from build123d import *

# Parameters (mm, degrees)
DODANIE_WYCI_GNI_CIE1_DEPTH = 26.5
SZKIC2_W                    = 110
SZKIC2_H                    = 20.5
WYTNIJ_WYCI_GNI_CIE1_DEPTH  = 30
SZKIC4_W                    = 20.5
SZKIC4_H                    = 25
WYTNIJ_WYCI_GNI_CIE3_DEPTH  = 3
SZKIC5_R                    = 1.6
WYTNIJ_WYCI_GNI_CIE4_DEPTH  = 135.815614823
FILLET1_R                   = 3


with BuildPart() as part:
    # Szkic1 → Dodanie-wyciągnięcie1 (new body)
    with BuildSketch(Plane.XY):
        Polygon((0, 0), (116, 0), (116, 28), (128, 28), (128, 33), (-12, 33), (-12, 28), (0, 28), align=None)
    extrude(amount=DODANIE_WYCI_GNI_CIE1_DEPTH)

    # Szkic2 → Wytnij-wyciągnięcie1 (cut)
    with BuildSketch(Plane(origin=(0, 33, 0), x_dir=(1, 0, 0), z_dir=(0, 1, 0))):
        with Locations((58, -13.25)):
            Rectangle(SZKIC2_W, SZKIC2_H)
    extrude(amount=-WYTNIJ_WYCI_GNI_CIE1_DEPTH, mode=Mode.SUBTRACT)

    # Szkic4 → Wytnij-wyciągnięcie3 (cut)
    with BuildSketch(Plane.ZY):
        with Locations((13.25, 15.5)):
            Rectangle(SZKIC4_W, SZKIC4_H)
    extrude(amount=-WYTNIJ_WYCI_GNI_CIE3_DEPTH, mode=Mode.SUBTRACT)

    # Szkic5 → Wytnij-wyciągnięcie4 (cut, through all)
    with BuildSketch(Plane(origin=(0, 33, 0), x_dir=(1, 0, 0), z_dir=(0, 1, 0))):
        with Locations(Location((-7, -5, 0), (0, 0, 180))):
            Circle(SZKIC5_R)
        with Locations(Location((123, -5, 0), (0, 0, 180))):
            Circle(SZKIC5_R)
        with Locations(Location((123, -21.5, 0), (0, 0, 180))):
            Circle(SZKIC5_R)
        with Locations(Location((-7, -21.5, 0), (0, 0, 180))):
            Circle(SZKIC5_R)
    extrude(amount=-WYTNIJ_WYCI_GNI_CIE4_DEPTH, mode=Mode.SUBTRACT)

    # Fillet1
    fillet1_edges = [part.edges().sort_by_distance(p)[0] for p in [
        (128, 30.5, 26.5),
        (-12, 30.5, 26.5),
        (-12, 30.5, 0),
        (128, 30.5, 0),
    ]]
    fillet(fillet1_edges, radius=FILLET1_R)


solid = part.part
Input: part model. Units: mm. Frame: model coordinates. A direction names the side the tool comes from. Give positions to 0.01 mm unless a question says otherwise; leave off trailing zeros. Write each loop counter-clockwise with the first axis right and the second up, starting at its lowest first coordinate (ties: lowest second). Pieces come first, ordered by that corner, then holes.
Q1. First-contact query: P1, Ø4, axis at x = 123, z = 5, coming from the +Y side; P2, Ø3.5, axis at x = 124, z = 17, coming from the -Y side; P3, Ø8, axis at y = 7.5, z = 10, coming from the -X side; P4, Ø12, axis at y = 5, z = 5.5, coming from the +X side. Flat tips, straight axial feed; report the tip coordinate or a pass-through.
Q2. Section A-A, the plane x = -7. Output: boundary loops of the cut face in (y, z).
Q3. Material intervals for probe 1 along Z at (x, y) = (-7, 30.6); probe 2 along Z at (x, y) = (41.5, 29.5); probe 3 along Y at (x, z) = (83.5, 7.5), sorted ascending.
Q4. Section D-D, the plane x = 105. Output: boundary loops of the cut face in (y, z), plus the area to 4 significant figures.
Q5. Section B-B, the plane z = 17. Output: boundary loops of the cut face in (x, y).
Q6. Set-up query: faces 1 (the face through (127.1, 30.54, 0.86)), 2 (the face through (116, 14, 13)), 3 (the face through (0, 2.7, 14.2)), 4 (the face through (-5, 28, 13)), 5 (the face through (57, 17, 0)). Return all of +Z, -Z, +X, -X, +Y, -Y with unobstructed straight access to the full face (end or side cutting, diameter ignored); none if empty.
Q7. Pull-direction query (X, two-part tool) for faces 6 (the face through (57, 17, 26.5)), 7 (the face through (3, 31, 13)), 8 (the face through (128, 30, 13)); classes: pulls with the +X half, pulls with the -X half, needs draft (parallel to the pull), parting line crosses it, or undercut.
Q8. Section C-C, the plane y = 13. Output: boundary loops of the cut face in (x, z).
Filled in:
1. P1: stops at y = 33
1. P2: stops at y = 28
1. P3: stops at x = 113
1. P4: stops at x = 116
2. outline: (28, 0) - (33, 0) - (33, 3.4) - (28, 3.4) - close; (28, 6.6) - (33, 6.6) - (33, 19.9) - (28, 19.9) - close; (28, 23.1) - (33, 23.1) - (33, 26.5) - (28, 26.5) - close
3. probe 1: z = 0 to 3.4, 6.6 to 19.9, 23.1 to 26.5
3. probe 2: z = 0 to 3, 23.5 to 26.5
3. probe 3: y = 0 to 3
4. outline: (0, 0) - (33, 0) - (33, 3) - (3, 3) - (3, 23.5) - (33, 23.5) - (33, 26.5) - (0, 26.5) - close
4. area: 259.5 mm2
5. outline: (-12, 28) - (3, 28) - (3, 33) - (-12, 33) - close; (0, 0) - (116, 0) - (116, 28) - (128, 28) - (128, 33) - (113, 33) - (113, 3) - (0, 3) - close
6. face 1: -Z, +X, +Y, -Y
6. face 2: +Z, -Z, +X, -Y
6. face 3: +Z, -Z, -X, -Y
6. face 4: -X
6. face 5: -Z, +X, -X, +Y, -Y
7. face 6: needs draft
7. face 7: undercut
7. face 8: pulls with the +X half
8. outline: (0, 0) - (116, 0) - (116, 26.5) - (0, 26.5) - (0, 23.5) - (113, 23.5) - (113, 3) - (0, 3) - close
